Verification items for the finished model (mm, model axes). A direction names the side the tool comes from. Round coordinates to 2 decimals unless told otherwise and drop trailing zeros. Loops run counter-clockwise (first coordinate to the right, second up) from the corner with the lowest first, then second, coordinate; pieces in that order, holes last.
from build123d import *

# Parameters (mm, degrees)
F0_W     = 50.8
F0_H     = 50.8
F1_DEPTH = 7.62
F2_T     = -2.54
F5_DEPTH = 25.4
F7_R     = 1.27
F7_W     = 8.9154
F7_H     = 1.27
F8_DEPTH = 4.572


with BuildPart() as f1:
    # F0 (on Top) → F1 (new body)
    with BuildSketch(Plane.XY):
        with Locations((25.4, 25.4)):
            Rectangle(F0_W, F0_H)
    extrude(amount=F1_DEPTH)

    # F2
    f2_openings = [f1.faces().sort_by_distance(p)[0] for p in [
        (25.4, 25.4, 7.62),
    ]]
    offset(amount=F2_T, openings=f2_openings)

    # F4 (on face) → F5 (cut)
    with BuildSketch(Plane.XY.offset(2.54)):
        with BuildLine():
            ThreePointArc((3.7855220646, 5.0770083749), (4.1574964525, 4.1789827628), (5.0555220646, 3.8070083749))
            Line((5.0555220646, 3.8070083749), (5.0555220646, 5.0770083749))
            Line((5.0555220646, 5.0770083749), (3.7855220646, 5.0770083749))
        make_face()
        with BuildLine():
            Line((5.0555220646, 5.0770083749), (5.0555220646, 3.8070083749))
            ThreePointArc((5.0555220646, 3.8070083749), (5.9535476767, 4.1789827628), (6.3255220646, 5.0770083749))
            ThreePointArc((6.3255220646, 5.0770083749), (5.0555220646, 6.3470083749), (3.7855220646, 5.0770083749))
            Line((3.7855220646, 5.0770083749), (5.0555220646, 5.0770083749))
        make_face()
    extrude(amount=-F5_DEPTH, mode=Mode.SUBTRACT)

    # F7 (on face) → F8 (join)
    with BuildSketch(Plane.XY.offset(2.54)):
        Polygon((48.26, 2.54), (48.26, 48.26), (2.54, 48.26), (2.54, 2.54), (7.62, 2.54), align=None)
        with Locations((10.8913211152, 27.047118172)):
            Circle(F7_R, mode=Mode.SUBTRACT)
        with Locations((34.3299443565, 37.2895654833)):
            Rectangle(F7_W, F7_H, mode=Mode.SUBTRACT)
    extrude(amount=F8_DEPTH)


solid = f1.part
1. Gauge pin test, flat ends, axial feed: P1, Ø2, axis at x = 10.89, y = 27.05, coming from the +Z side; P2, Ø2, axis at x = 11.5, y = 27, coming from the +Z side. Record the tip position at first contact, or that the pin passes through.
2. Release check for a two-part mould opening along X. For faces 4 (the face through (34, 36.655, 5)), 5 (the face through (0, 25, 4)), 6 (the face through (23, 1, 7.62)) record: released by +X, released by -X, zero draft, split by the parting line, or undercut.
3. Section check A-A (x = 40). Enter the section's corners in (y, z).
4. Scan lines: L1, parallel to Z at x = 22, y = 38.5; L2, parallel to Y at x = 10, z = 6.5. Record each from-to range of solid material in increasing order.
5. Tool access check on faces 1 (the face through (34, 37.925, 5)), 2 (the face through (5, 5, 2.54)), 3 (the face through (25, 26, 0)). Record the directions out of +Z, -Z, +X, -X, +Y, -Y that give a thin tool (end or side, any length) a straight path to the whole face; none if there is none.
Taken from the geometry:
1. P1: stops at z = 2.54
1. P2: stops at z = 7.11
2. face 4: undercut
2. face 5: released by -X
2. face 6: zero draft
3. outline: (0, 0) - (50.8, 0) - (50.8, 7.62) - (48.26, 7.62) - (48.26, 7.11) - (2.54, 7.11) - (2.54, 7.62) - (0, 7.62) - close
4. L1: z = 0 to 7.11
4. L2: y = 0 to 26.14, 27.95 to 50.8
5. face 1: +Z
5. face 2: -Z
5. face 3: -Z, +X, -X, +Y, -Y
